```python
from build123d import *

# Parameters (mm, degrees)
SKETCH_R                       = 2.25
SKETCH_R_2                     = 1.75
PAD_DEPTH                      = 12
POCKET_DEPTH                   = 2
SKETCH002_R                    = 2.25
POCKET002_DEPTH                = 20.001
PART_MIRRORING_PLACEMENT_ANGLE = 180
SKETCH003_R                    = 3
POCKET003_DEPTH                = 8
SKETCH004_R                    = 3.75
POCKET004_DEPTH                = 10


with BuildPart() as pocket002:
    # Sketch → Pad (new body)
    with BuildSketch(Plane.XY):
        Polygon((0, -20), (40, -20), (40, 20), (-20, 20), (-20, 0), (0, 0), align=None)
        with Locations((15, 8)):
            Circle(SKETCH_R, mode=Mode.SUBTRACT)
        with Locations((10, -10)):
            Circle(SKETCH_R, mode=Mode.SUBTRACT)
        with Locations((35, 15)):
            Circle(SKETCH_R_2, mode=Mode.SUBTRACT)
        with Locations((25, -10)):
            Circle(SKETCH_R, mode=Mode.SUBTRACT)
    extrude(amount=PAD_DEPTH)

    # Sketch001 → Pocket (cut)
    with BuildSketch(Plane.XY.offset(12)):
        with BuildLine():
            Line((46, 10), (26, 10))
            ThreePointArc((26, 10), (22.778175, 17.778175), (15, 21))
            Line((15, 21), (0, 21))
            Line((0, 21), (0, -23))
            Line((0, -23), (46, -23))
            Line((46, -23), (46, -12))
            Line((25.538775, -14.46763), (46, -12))
            ThreePointArc((25.538775, -5.53237), (20.5, -10), (25.538775, -14.46763))
            Line((25.538775, -5.53237), (46, -8))
            Line((46, -8), (46, 10))
        make_face()
    extrude(amount=-POCKET_DEPTH, mode=Mode.SUBTRACT)

    # Sketch002 → Pocket002 (cut, through all)
    with BuildSketch(Plane.XZ):
        with Locations((-10, 6)):
            Circle(SKETCH002_R)
    extrude(amount=-POCKET002_DEPTH, mode=Mode.SUBTRACT)


with BuildPart() as pocket004:
    # Part__Mirroring: instance of Pocket002
    add(pocket002.part.mirror(Plane(origin=(0, 0, 0), x_dir=(0, 1, 0), z_dir=(0, 0, 1))))


with BuildPart() as pocket004_1:
    # Part__Mirroring placement: moved
    add(pocket004.part.rotate(Axis((0, 0, 0), (1, 0, 0)), PART_MIRRORING_PLACEMENT_ANGLE))

    # Sketch003 → Pocket003 (cut)
    with BuildSketch(Plane(origin=(0, 0, 0), x_dir=(1, 0, 0), z_dir=(0, 0, -1))):
        with Locations((35, 15)):
            Circle(SKETCH003_R)
    extrude(amount=-POCKET003_DEPTH, mode=Mode.SUBTRACT)

    # Sketch004 → Pocket004 (cut)
    with BuildSketch(Plane(origin=(0, -20, 0), x_dir=(-1, 0, 0), z_dir=(0, -1, 0))):
        with Locations((10, -6)):
            Circle(SKETCH004_R)
    extrude(amount=-POCKET004_DEPTH, mode=Mode.SUBTRACT)


with BuildPart() as part_mirroring001:
    # Part__Mirroring001: instance of Pocket004
    add(pocket004_1.part.mirror(Plane(origin=(0, 0, 0), x_dir=(0, -1, 0), z_dir=(1, 0, 0))))


solid = part_mirroring001.part
```
The listing builds one solid part. Answer for the finished solid, in the listing's coordinates (mm). A direction names the side the tool comes from. Give positions to 0.01 mm unless a question says otherwise; leave off trailing zeros. Loops run counter-clockwise (first coordinate to the right, second up) from the corner with the lowest first, then second, coordinate; pieces in that order, holes last. Notation, with made-up numbers: (74.25, 25.25) - (104.25, 25.25) arc R20 cw to (104.25, 49.25) - close; hole circle Ø8 at (-35.75, 73). An arc over 180 degrees is marked (long way). Return JSON: item names as keys, results as strings. Group by question number.
1. Find section A-A (y = 10). Write down the section's boundary in (x, z).
2. Straight lines are drawn through the part: line 1 (Y direction, x = -35, z = 4); line 2 (Z direction, x = 10, y = -15.75); line 3 (Y direction, x = -35, z = 9.65). For each, find the intervals that lie inside material, in ascending order. Write a range as [from, to].
3. Find section B-B (x = -10). Write down the section's boundary in (y, z).
4. Given pin 1 Ø1.8 at (x, y) = (-35, -15) entering from -Z; pin 2 Ø6 at (x, z) = (10, 6) entering from +Y; pin 3 Ø0.6 at (x, z) = (-32.5, 10.5) entering from +Y; pin 4 Ø2 at (x, z) = (8.5, 4) entering from -Y, each flat-ended and moving along its own axis, determine where each tip first touches the part or whether it passes through.
5. Which of the six approach directions +Z, -Z, +X, -X, +Y, -Y give full straight-line access (tool end or side, diameter ignored) to faces 5 (the cylindrical face through (-24.305, -15.867, 11.014)), 6 (the flat face through (12.4, 0, 5.9)), 7 (the flat face through (0, -10, 11)), 8 (the flat face through (-32.668, 13.608, 11.014))?
6. Find section C-C (y = -15). Write down the section's boundary in (x, z).
7. Find section D-D (y = -3). Write down the section's boundary in (x, z).
8. Determine the mould class of faces 1 (the flat face through (12, -10, 8)), 2 (the cylindrical face through (-8.34, 8.48, 4.93)), 3 (the cylindrical face through (-32, -15, 4)), 4 (the flat face through (20, -10, 6)) for opening direction Y: pulls with the +Y half, pulls with the -Y half, needs draft (parallel to the pull), parting line crosses it, or undercut.
Verdict:
{
 "1": {"outline": "(-40, 0) - (-27.25, 0) - (-27.25, 12) - (-40, 12) - close; (-22.75, 0) - (-12.25, 0) - (-12.25, 10) - (-20.5, 10) - (-20.5, 12) - (-22.75, 12) - close; (-7.75, 0) - (0, 0) - (0, 10) - (-7.75, 10) - close"},
 "2": {"line 1": "y = [-20, -18], [-12, 20]", "line 2": "z = [0, 2.25], [9.75, 12]", "line 3": "y = [-20, -16.75], [-13.25, 20]"},
 "3": {"outline": "(-20, 0) - (7.75, 0) - (7.75, 10) - (-20, 10) - close; (12.25, 0) - (20, 0) - (20, 10) - (12.25, 10) - close"},
 "4": {"pin 1": "passes through", "pin 2": "stops at y = 0", "pin 3": "stops at y = 13.66", "pin 4": "stops at y = -10"},
 "5": {"face 5": "+Z", "face 6": "+Z, -Z, +X, +Y", "face 7": "+Z, +Y, -Y", "face 8": "+Z, -X, +Y"},
 "6": {"outline": "(-40, 0) - (-38, 0) - (-38, 8) - (-36.75, 8) - (-36.75, 12) - (-40, 12) - close; (-33.25, 8) - (-32, 8) - (-32, 0) - (20, 0) - (20, 12) - (0, 12) - (0, 10) - (-24.8, 10) - (-24.8, 12) - (-33.25, 12) - close; hole circle Ø7.5 at (10, 6)"},
 "7": {"outline": "(-40, 0) - (20, 0) - (20, 12) - (0, 12) - (0, 10) - (-40, 10) - close; hole circle Ø4.5 at (10, 6)"},
 "8": {"face 1": "pulls with the -Y half", "face 2": "undercut", "face 3": "undercut", "face 4": "needs draft"}
}
